Work out the finished part from the listing and answer in its coordinate system (mm). A direction names the side the tool comes from. Coordinates: 2 decimals unless noted, no trailing zeros. Order: outer loops, then holes, each group sorted by start corner. A loop starts at its lowest first (then second) coordinate and runs counter-clockwise, first axis right, second up. Notation, with made-up numbers: M -6.5,-9.75 L 8.5,-9.75 A38 cw 8.5,28.25 Z; hole C -21,36 d6. An arc over 180 degrees is marked long. Use a Markdown table: item, result.
from build123d import *

# Parameters (mm, degrees)
SKETCH_1_R          = 4
EXTRUDE_1_DEPTH     = 30
SKETCH_3_R          = 1.7
CUT_EXTRUDE_1_DEPTH = 30
SKETCH_4_R          = 2
CUT_EXTRUDE_2_DEPTH = 6


with BuildPart() as part:
    # 草图1 → 凸台-拉伸1 (new body)
    with BuildSketch(Plane.XY):
        Polygon((-17, -7), (-7, -7), (-5, -11), (5, -11), (7, -7), (17, -7), (17, 11), (-17, 11), align=None)
        Circle(SKETCH_1_R, mode=Mode.SUBTRACT)
    extrude(amount=EXTRUDE_1_DEPTH)

    # 草图3 → 切除-拉伸1 (cut)
    with BuildSketch(Plane(origin=(0, 11, 0), x_dir=(1, 0, 0), z_dir=(0, 1, 0))):
        with Locations(Location((12, -6, 0), (0, 0, 270))):
            Circle(SKETCH_3_R)
        with Locations(Location((-12, -6, 0), (0, 0, 270))):
            Circle(SKETCH_3_R)
        with Locations(Location((-12, -24, 0), (0, 0, 270))):
            Circle(SKETCH_3_R)
        with Locations(Location((12, -24, 0), (0, 0, 270))):
            Circle(SKETCH_3_R)
    extrude(amount=-CUT_EXTRUDE_1_DEPTH, mode=Mode.SUBTRACT)

    # 草图4 → 切除-拉伸2 (cut)
    with BuildSketch(Plane.XZ.offset(7)):
        with Locations(Location((-12, 24, 0), (0, 0, 270))):
            Circle(SKETCH_4_R)
        with Locations(Location((12, 24, 0), (0, 0, 270))):
            Circle(SKETCH_4_R)
        with Locations(Location((12, 6, 0), (0, 0, 270))):
            Circle(SKETCH_4_R)
        with Locations(Location((-12, 6, 0), (0, 0, 270))):
            Circle(SKETCH_4_R)
    extrude(amount=-CUT_EXTRUDE_2_DEPTH, mode=Mode.SUBTRACT)


solid = part.part
(1) A cutting plane is placed at C-C (x = 0). Determine the outline of the cut face in (y, z).
Conclusion:
| item | result |
|---|---|
| outline | M -11,0 L -4,0 L -4,30 L -11,30 Z; M 4,0 L 11,0 L 11,30 L 4,30 Z |
(2) Determine the mould class of faces 1 (the flat face through (-17, 2, 15)), 2 (the cylindrical face through (-13.66, 5.08, 5.63)), 3 (the cylindrical face through (-10, -4, 6)), 4 (the flat face through (0, 5, 0)) for opening direction X: pulls with the +X half, pulls with the -X half, needs draft (parallel to the pull), parting line crosses it, or undercut.
Conclusion:
| item | result |
|---|---|
| face 1 | pulls with the -X half |
| face 2 | undercut |
| face 3 | undercut |
| face 4 | needs draft |
(3) Given P1, Ø4.5, axis at x = -11.5, z = 6, coming from the -Y side; P2, Ø1.2, axis at x = 12, z = 24.5, coming from the -Y side, each flat-ended and moving along its own axis, determine where each tip first touches the part or whether it passes through.
Conclusion:
| item | result |
|---|---|
| P1 | y = -7 |
| P2 | through |
(4) A cutting plane is placed at D-D (x = -12). Determine the outline of the cut face in (y, z), then the cut area to 3 significant figures.
Conclusion:
| item | result |
|---|---|
| outline | M -7,0 L 11,0 L 11,4.3 L -1,4.3 L -1,4 L -7,4 Z; M -7,8 L -1,8 L -1,7.7 L 11,7.7 L 11,22.3 L -1,22.3 L -1,22 L -7,22 Z; M -7,26 L -1,26 L -1,25.7 L 11,25.7 L 11,30 L -7,30 Z |
| area | 410 mm2 |
(5) Straight lines are drawn through the part: L1, parallel to X at y = 10.25, z = 6.5; L2, parallel to Y at x = 0, z = 16.75; L3, parallel to Y at x = -9, z = 1.5. For each, find the intervals that lie inside material, in ascending order.
Conclusion:
| item | result |
|---|---|
| L1 | -17 to -13.62, -10.38 to 10.38, 13.62 to 17 |
| L2 | -11 to -4, 4 to 11 |
| L3 | -7 to 11 |
(6) A cutting plane is placed at A-A (y = 0). Determine the outline of the cut face in (x, z), then the cut area to 3 significant figures.
Conclusion:
| item | result |
|---|---|
| outline | M -17,0 L -4,0 L -4,30 L -17,30 Z; M 4,0 L 17,0 L 17,30 L 4,30 Z; hole C -12,6 d3.4; hole C -12,24 d3.4; hole C 12,6 d3.4; hole C 12,24 d3.4 |
| area | 744 mm2 |
(7) Which of the six approach directions +Z, -Z, +X, -X, +Y, -Y give full straight-line access (tool end or side, diameter ignored) to faces 5 (the cylindrical face through (14, -4, 6)), 6 (the flat face through (17, 2, 15))?
Conclusion:
| item | result |
|---|---|
| face 5 | -Y |
| face 6 | +Z, -Z, +X, +Y, -Y |
(8) A cutting plane is placed at B-B (z = 6). Determine the outline of the cut face in (x, y).
Conclusion:
| item | result |
|---|---|
| outline | M -17,-7 L -14,-7 L -14,-1 L -13.7,-1 L -13.7,11 L -17,11 Z; M -10.3,-1 L -10,-1 L -10,-7 L -7,-7 L -5,-11 L 5,-11 L 7,-7 L 10,-7 L 10,-1 L 10.3,-1 L 10.3,11 L -10.3,11 Z; M 13.7,-1 L 14,-1 L 14,-7 L 17,-7 L 17,11 L 13.7,11 Z; hole C 0,0 d8 |
